The model under review builds one solid part; all positions refer to its coordinate system, in mm. Face numbers are marked on the shaded views. A direction names the side the tool comes from. Give positions to 0.01 mm unless a question says otherwise; leave off trailing zeros. Order: outer loops, then holes, each group sorted by start corner. A loop starts at its lowest first (then second) coordinate and runs counter-clockwise, first axis right, second up. Notation, with made-up numbers: (44.25, 32) - (74.25, 32) arc R6 ccw to (74.25, 37) - close; hole circle Ø5 at (80.25, -19.75). An arc over 180 degrees is marked (long way). Answer as CSV lines item,"result". Start each with the question number.
Autodesk Inventor part; units mm, degrees
ref_plane "Work Plane1" through (-12.875, -12.875, 4.75) normal (0, 0, -1) x (0, 1, 0)
ref_plane "YZ Plane" through (0, 0, 0) normal (1, 0, 0) x (0, 1, 0)
ref_plane "XZ Plane" through (0, 0, 0) normal (0, 1, 0) x (-1, 0, 0)
sketch "Sketch1" plane through (0, 0, 0) normal (0, 0, 1) x (1, 0, 0)
  line L0 (1.9666, 1.85) -> (-1.9666, 1.85) construction
  arc A0 (-1.9666, 1.85) -> (-1.9666, -1.85) centre (0, 0) ccw construction
  arc A1 (1.9666, -1.85) -> (1.9666, 1.85) centre (0, 0) ccw construction
  line L1 (-1.9666, -1.85) -> (1.9666, -1.85) construction
  circle A2 centre (0, 0) radius 4.7
  arc A3 (-2.0304, 2) -> (-2.0304, -2) centre (0, 0) ccw
  line L2 (-2.0304, 2) -> (2.0304, 2)
  line L3 (-2.0304, -2) -> (2.0304, -2)
  arc A4 (2.0304, -2) -> (2.0304, 2) centre (0, 0) ccw
  dimension "d0" = 2
  dimension "d6" = 0.15
  dimension "d7" = 0.15
ref_plane "Work Plane1" through (-12.875, -12.875, 4.75) normal (0, 0, -1) x (0, 1, 0)
extrude "Extrusion1" add sketch "Sketch1" along normal up to surface (4.75 mm away)
properties part number "TTencoderspacer"
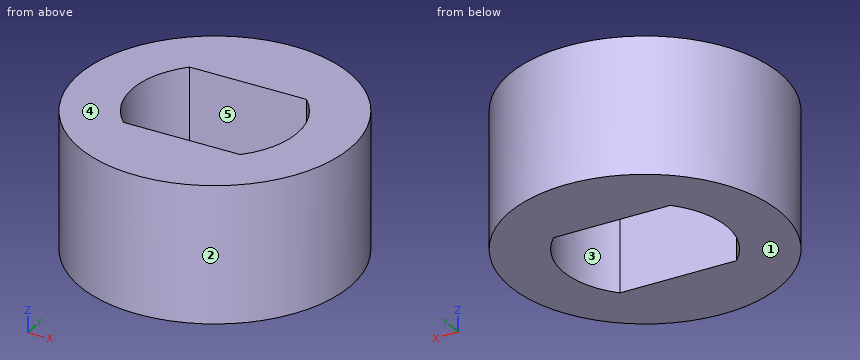
Item 1: Take a section at A-A on x = 0. Write out the cut boundary in (y, z).
Item 2: Take a section at D-D on x = 3.5. Write out the cut boundary in (y, z).
Item 3: Take a section at B-B on y = 0. Write out the cut boundary in (x, z).
Item 4: Mouldability with a two-part tool opening along Y and no side actions: class the marked faces 1, 2 and 3 as released by +Y, released by -Y, zero draft, split by the parting line, or undercut.
Item 5: Clearance check with a flat-ended pin moving along its axis: pin 1 (2 mm diameter, centred on y = 2.5, z = 3, fed in from +X). State where the tip first meets the part, or that it passes through.
Item 6: For line 1 along Y through (x, z) = (-2, 3.8); line 2 along Y through (x, z) = (0.75, 1.1); line 3 along X through (y, z) = (-0.75, 0.95), list the stretches that pass through material, from the lowest coordinate up.
Item 7: Take a section at C-C on z = 4.2. Write out the cut boundary in (x, y), and give its area (3 significant figures).
Item 8: Machinability: for the marked faces 4 and 5, which of the approach directions +Z, -Z, +X, -X, +Y, -Y give a long, thin tool a straight path to every point of the face, cutting with its end or side? Answer none if there is none.
Data:
1,outline,"(-4.7, 0) - (-2, 0) - (-2, 4.75) - (-4.7, 4.75) - close; (2, 0) - (4.7, 0) - (4.7, 4.75) - (2, 4.75) - close"
2,outline,"(-3.14, 0) - (3.14, 0) - (3.14, 4.75) - (-3.14, 4.75) - close"
3,outline,"(-4.7, 0) - (-2.85, 0) - (-2.85, 4.75) - (-4.7, 4.75) - close; (2.85, 0) - (4.7, 0) - (4.7, 4.75) - (2.85, 4.75) - close"
4,face 1,"zero draft"
4,face 2,"split by the parting line"
4,face 3,"undercut"
5,pin 1,"stops at x = 4.45"
6,line 1,"y = -4.25 to -2, 2 to 4.25"
6,line 2,"y = -4.64 to -2, 2 to 4.64"
6,line 3,"x = -4.64 to -2.75, 2.75 to 4.64"
7,outline,"circle Ø9.4 at (0, 0); hole (-2.03, -2) - (2.03, -2) arc R2.85 ccw to (2.03, 2) - (-2.03, 2) arc R2.85 ccw to start"
7,area,"48.6 mm^2"
8,face 4,"+Z, +X, -X, +Y, -Y"
8,face 5,"+Z, -Z"
